Part model, mm, in its own coordinate system. A direction names the side the tool comes from. Coordinates: 2 decimals unless noted, no trailing zeros. Loops run counter-clockwise (first coordinate to the right, second up) from the corner with the lowest first, then second, coordinate; pieces in that order, holes last. Notation, with made-up numbers: M 6,58.25 L 26,58.25 A21 ccw 26,94.25 Z; hole C 72.5,48.5 d11. An arc over 180 degrees is marked long. Use a Markdown table: item, result. Add a question column.
1) Wall check: probe 1 along X at (y, z) = (13.5, 17); probe 2 along Z at (x, y) = (15, 2.25); probe 3 along Z at (x, y) = (15, 2.5). Give the ranges that are in metal, low to high. Write a range as from..to.
2) Pull direction X, two halves, no side cores. Call faces 3 (the cylindrical face through (6.85, 2.62, 71.04)), 4 (the flat face through (19, 20, 70)): released by +X, released by -X, zero draft, split by the parting line, or undercut.
3) Band-saw the part on B-B (z = 81). State how many separate pieces and enclosed holes the cut face has, plus the area to 3 significant figures.
4) Band-saw the part on A-A (y = 13.5). List the corners of the cut face in (x, z).
5) Tool access for faces 1 (the flat face through (17, 10, 69)), 2 (the flat face through (110, 20, 67)): list every direction of +Z, -Z, +X, -X, +Y, -Y with a clear straight run to the whole face (end or side of a thin tool).
6) Pin check, flat tips, straight feed: pin 1 Ø1 at (x, z) = (48, 41) entering from +Y; pin 2 Ø5 at (x, z) = (5, 71.13) entering from +Y; pin 3 Ø8 at (x, y) = (34.5, 12.5) entering from -Z. Stop position of each tip, or through.
from build123d import *

# Parameters (mm, degrees)
SKETCH3_R           = 1.85
CUT_EXTRUDE1_DEPTH  = 155.06371723
SKETCH4_R           = 3.85
SKETCH4_R_2         = 1.85
BOSS_EXTRUDE1_DEPTH = 10


with BuildPart() as part:
    # Sketch1 → Loft1 section 0
    with BuildSketch(Plane(origin=(0, 0, 0), x_dir=(1, 0, 0), z_dir=(0, 1, 0))):
        with BuildLine():
            Line((0, 0), (127.35007717, 0))
            Line((127.35007717, 0), (127.35007717, -86.125413014))
            Line((127.35007717, -86.125413014), (0, -86.125413014))
            Line((0, -86.125413014), (0, 0))
        make_face()
    # Sketch2 → Loft1 section 1
    with BuildSketch(Plane(origin=(0, 10, 0), x_dir=(1, 0, 0), z_dir=(0, 1, 0))):
        with BuildLine():
            Line((10, -10), (10, -76.125413014))
            Line((10, -76.125413014), (117.35007717, -76.125413014))
            Line((117.35007717, -76.125413014), (117.35007717, -10))
            Line((117.35007717, -10), (10, -10))
        make_face()
    loft()

    # Sketch3 → Cut-Extrude1 (cut, through all)
    with BuildSketch(Plane.XZ):
        with Locations(Location((5, 15, 0), (0, 0, 270))):
            Circle(SKETCH3_R)
        with Locations(Location((5, 71.125413014, 0), (0, 0, 180))):
            Circle(SKETCH3_R)
        with Locations(Location((122.35007717, 71.125413014, 0), (0, 0, 270))):
            Circle(SKETCH3_R)
        with Locations((122.35007717, 15)):
            Circle(SKETCH3_R)
        with Locations(Location((15, 5, 0), (0, 0, 270))):
            Circle(SKETCH3_R)
        with Locations(Location((15, 81.125413014, 0), (0, 0, 270))):
            Circle(SKETCH3_R)
        with Locations(Location((112.35007717, 81.125413014, 0), (0, 0, 90))):
            Circle(SKETCH3_R)
        with Locations(Location((112.35007717, 5, 0), (0, 0, 270))):
            Circle(SKETCH3_R)
    extrude(amount=-CUT_EXTRUDE1_DEPTH, mode=Mode.SUBTRACT)

    # Sketch4 → Boss-Extrude1 (add)
    # profile 1 of 4: a face of its own
    with BuildSketch(Plane(origin=(0, 10, 0), x_dir=(1, 0, 0), z_dir=(0, 1, 0))):
        with Locations(Location((110.35007717, -69.125413014, 0), (0, 0, 270))):
            Circle(SKETCH4_R)
        with Locations(Location((110.35007717, -69.125413014, 0), (0, 0, 270))):
            Circle(SKETCH4_R_2, mode=Mode.SUBTRACT)
    # profile 2 of 4: a face of its own
    with BuildSketch(Plane(origin=(0, 10, 0), x_dir=(1, 0, 0), z_dir=(0, 1, 0))):
        with Locations(Location((110.35007717, -17, 0), (0, 0, 90))):
            Circle(SKETCH4_R)
        with Locations(Location((110.35007717, -17, 0), (0, 0, 90))):
            Circle(SKETCH4_R_2, mode=Mode.SUBTRACT)
    # profile 3 of 4: a face of its own
    with BuildSketch(Plane(origin=(0, 10, 0), x_dir=(1, 0, 0), z_dir=(0, 1, 0))):
        with Locations(Location((17, -17, 0), (0, 0, 270))):
            Circle(SKETCH4_R)
        with Locations(Location((17, -17, 0), (0, 0, 270))):
            Circle(SKETCH4_R_2, mode=Mode.SUBTRACT)
    # profile 4 of 4: a face of its own
    with BuildSketch(Plane(origin=(0, 10, 0), x_dir=(1, 0, 0), z_dir=(0, 1, 0))):
        with Locations(Location((17, -69.125413014, 0), (0, 0, 90))):
            Circle(SKETCH4_R)
        with Locations(Location((17, -69.125413014, 0), (0, 0, 90))):
            Circle(SKETCH4_R_2, mode=Mode.SUBTRACT)
    extrude(amount=BOSS_EXTRUDE1_DEPTH)


solid = part.part
Entries:
| question | item | result |
|---|---|---|
| 1 | probe 1 | 13.15..15.15, 18.85..20.85, 106.5..108.5, 112.2..114.2 |
| 1 | probe 2 | 2.25..3.15, 6.85..79.28, 82.98..83.88 |
| 1 | probe 3 | 2.5..3.15, 6.85..79.28, 82.98..83.63 |
| 2 | face 3 | undercut |
| 2 | face 4 | zero draft |
| 3 | separate pieces | 3 |
| 3 | enclosed holes | 0 |
| 3 | area | 589 mm2 |
| 4 | outline | C 17,17 d7.7; C 17,69.13 d7.7; C 110.35,17 d7.7; C 110.35,69.13 d7.7; hole C 17,17 d3.7; hole C 17,69.13 d3.7; hole C 110.35,17 d3.7; hole C 110.35,69.13 d3.7 |
| 5 | face 1 | +Y |
| 5 | face 2 | +Z, -Z, +X, -X, +Y |
| 6 | pin 1 | y = 10 |
| 6 | pin 2 | y = 7.5 |
| 6 | pin 3 | z = 8.5 |
